The model under review builds one solid part; all positions refer to its coordinate system, in mm. A direction names the side the tool comes from. Coordinates: 2 decimals unless noted, no trailing zeros. Order: outer loops, then holes, each group sorted by start corner. A loop starts at its lowest first (then second) coordinate and runs counter-clockwise, first axis right, second up. Notation, with made-up numbers: M 34.5,-9 L 83.5,-9 A17 cw 83.5,10 Z; hole C 71,-19.5 d5. An arc over 180 degrees is marked long. Write each question's results on one line, items separated by ' | '.
from build123d import *

# Parameters (mm, degrees)
F0_R          = 3.5
F0_R_2        = 2.5
F1_DEPTH      = 8.5
F1_DEPTH_BACK = 8.5
F3_DEPTH      = 17.001


with BuildPart() as f1:
    # F0 (on Front) → F1 (new body, two sides)
    with BuildSketch(Plane.XZ) as f1_sk:
        Circle(F0_R)
        Circle(F0_R_2, mode=Mode.SUBTRACT)
    extrude(amount=F1_DEPTH)
    extrude(f1_sk.sketch, amount=-F1_DEPTH_BACK)

    # F2 (on face) → F3 (cut, through all)
    with BuildSketch(Plane.XZ.offset(8.5)):
        with BuildLine():
            Line((2.5, 0), (-2.5, 0))
            ThreePointArc((-2.5, 0), (0, -2.5), (2.5, 0))
        make_face()
        with BuildLine():
            ThreePointArc((0, -3.5), (-1.355874, -3.226702), (-2.5, -2.44949))
            Line((-2.5, -2.44949), (-2.5, -3.5))
            Line((-2.5, -3.5), (0, -3.5))
        make_face()
        with BuildLine():
            ThreePointArc((2.5, 0), (0, -2.5), (-2.5, 0))
            Line((-2.5, 0), (-2.5, -2.44949))
            ThreePointArc((-2.5, -2.44949), (-1.355874, -3.226702), (0, -3.5))
            ThreePointArc((0, -3.5), (1.355874, -3.226702), (2.5, -2.44949))
            Line((2.5, -2.44949), (2.5, 0))
        make_face()
        with BuildLine():
            Line((2.5, -3.5), (2.5, -2.44949))
            ThreePointArc((2.5, -2.44949), (1.355874, -3.226702), (0, -3.5))
            Line((0, -3.5), (2.5, -3.5))
        make_face()
    extrude(amount=-F3_DEPTH, mode=Mode.SUBTRACT)


solid = f1.part
1) The part is to be moulded in two halves that separate along X. For faces 1 (the flat face through (2.5, 0, -1)), 2 (the cylindrical face through (0.1, -0.1, 3.5)), 3 (the flat face through (-1, -8.5, 3)), say which applies: pulls with the +X half, pulls with the -X half, needs draft (parallel to the pull), parting line crosses it, or undercut.
Solutions:
face 1: undercut | face 2: parting line crosses it | face 3: needs draft
2) Take a section at C-C on z = -1.35. State the section outline as (x, y) points, plus the area to 3 significant figures.
Solutions:
outline: M -3.23,-8.5 L -2.5,-8.5 L -2.5,8.5 L -3.23,8.5 Z; M 2.5,-8.5 L 3.23,-8.5 L 3.23,8.5 L 2.5,8.5 Z | area: 24.8 mm2
3) To check wall thickness, follow line 1 along X through (y, z) = (-1.5, 1.9); line 2 along X through (y, z) = (-2.75, -1.4); line 3 along Z through (x, y) = (1.75, 2.25). State the ranges of each line that lie inside material, in increasing order.
Solutions:
line 1: -2.94 to -1.62, 1.62 to 2.94 | line 2: -3.21 to -2.5, 2.5 to 3.21 | line 3: 1.79 to 3.03
4) Take a section at D-D on y = 5.5. State the section outline as (x, z) points.
Solutions:
outline: M -2.5,-2.45 L -2.5,0 A2.5 cw 2.5,0 L 2.5,-2.45 A3.5 ccw long Z
5) Take a section at A-A on z = 0.65. State the section outline as (x, y) points.
Solutions:
outline: M -3.44,-8.5 L -2.41,-8.5 L -2.41,8.5 L -3.44,8.5 Z; M 2.41,-8.5 L 3.44,-8.5 L 3.44,8.5 L 2.41,8.5 Z
6) Take a section at B-B on x = 0. State the section outline as (y, z) points.
Solutions:
outline: M -8.5,2.5 L 8.5,2.5 L 8.5,3.5 L -8.5,3.5 Z
7) For faces 4 (the flat face through (-1, 8.5, 3)), 5 (the flat face through (-2.5, 0, -1)), list the 3-axis set-ups (+Z, -Z, +X, -X, +Y, -Y) from which the entire face can be reached by the end or side of a thin tool; tool diameter is ignored.
Solutions:
face 4: +Z, -Z, +X, -X, +Y | face 5: -Z, +Y, -Y
8) For pin 1 (3 mm diameter, centred on y = 4, z = -2, fed in from +X); pin 2 (1.2 mm diameter, centred on y = -2.5, z = -1.5, fed in from -X); pin 3 (1.5 mm diameter, centred on x = -1, z = -0.5, fed in from +Y); pin 4 (0.7 mm diameter, centred on y = -3.5, z = -1, fed in from +X), all flat-tipped, find the tip position at first contact; note any pin that passes through.
Solutions:
pin 1: x = 3.46 | pin 2: x = -3.38 | pin 3: through | pin 4: x = 3.44
